```python
from build123d import *

# Parameters (mm, degrees)
FILLET1_R  = 0.4
SKETCH2_W  = 16.4
SKETCH2_H  = 1.6
SLOT_DEPTH = 2.8


with BuildPart() as part:
    # BodySke → Base-Revolve (revolve)
    with BuildSketch(Plane.XY, mode=Mode.PRIVATE) as base_revolve_sk:
        with BuildLine():
            Line((4.8, 4), (4.8, 8.2))
            Line((4.8, 8.2), (4.79, 8.2))
            Line((4.79, 8.2), (1.7, 7.92966003))
            ThreePointArc((1.7, 7.92966003), (0.429774249, 4.054920104), (0, 0))
            Line((0, 0), (39.8, 0))
            Line((39.8, 0), (39.8, 4))
            Line((39.8, 4), (4.8, 4))
        make_face()
    revolve(base_revolve_sk.sketch.rotate(Axis((-25.4, 0, 0), (1, 0, 0)), 90), axis=Axis((-25.4, 0, 0), (1, 0, 0)))

    # Fillet1
    fillet1_edges = [part.edges().sort_by_distance(p)[0] for p in [
        (4.8, 0, -4),
    ]]
    fillet(fillet1_edges, radius=FILLET1_R)

    # Sketch2 → Slot (cut)
    with BuildSketch(Plane(origin=(0, 0, 0), x_dir=(0, 0, -1), z_dir=(1, 0, 0))):
        Rectangle(SKETCH2_W, SKETCH2_H)
    extrude(amount=SLOT_DEPTH, mode=Mode.SUBTRACT)


solid = part.part
```
Work out the finished part from the listing and answer in its coordinate system (mm). A direction names the side the tool comes from. Give positions to 0.01 mm unless a question says otherwise; leave off trailing zeros. Write each loop counter-clockwise with the first axis right and the second up, starting at its lowest first coordinate (ties: lowest second). Pieces come first, ordered by that corner, then holes.
(1) Which of the six approach directions +Z, -Z, +X, -X, +Y, -Y give full straight-line access (tool end or side, diameter ignored) to faces 4 (the cylindrical face through (22.258, 3.905, -0.867)), 5 (the flat face through (2.8, 0, 0))?
Final values:
face 4: +X
face 5: +Z, -Z, -X
(2) Flat-ended cylindrical pins translate along their axes: pin 1 Ø8 at (x, z) = (19, 4) entering from +Y; pin 2 Ø0.5 at (y, z) = (-0.5, -2.5) entering from -X; pin 3 Ø2 at (y, z) = (-5.5, -2.5) entering from -X. Find the tip coordinate at first contact, or state that the pin passes through.
Final values:
pin 1: stops at y = 4
pin 2: stops at x = 2.8
pin 3: stops at x = 0.67
(3) The mould has two halves that part along Y. Classify faces 1 (the conical face through (2.537, -2.404, 7.633)), 2 (the flat face through (2, -0.8, 0)), 3 (the flat face through (39.8, 0, 0)): pulls with the +Y half, pulls with the -Y half, needs draft (parallel to the pull), parting line crosses it, or undercut.
Final values:
face 1: parting line crosses it
face 2: undercut
face 3: needs draft
(4) Straight lines are drawn through the part: line 1 (X direction, y = -0.5, z = 2.75); line 2 (Y direction, x = 28, z = 0); line 3 (Y direction, x = 2, z = 7). For each, find the intervals that lie inside material, in ascending order.
Final values:
line 1: x = 2.8 to 39.8
line 2: y = -4 to 4
line 3: y = -3.78 to -0.8, 0.8 to 3.78
(5) The part is cut by section C-C on x = 34. Write down the section's boundary in (y, z).
Final values:
outline: circle Ø8 at (0, 0)
